Check sheet for the modelled part. Datum: model origin and axes. Units: mm. Round coordinates to 2 decimals unless told otherwise and drop trailing zeros. Loops run counter-clockwise (first coordinate to the right, second up) from the corner with the lowest first, then second, coordinate; pieces in that order, holes last. Notation, with made-up numbers: (5.5, -26) - (54.5, -26) arc R24 ccw to (54.5, 6) - close; hole circle Ø2 at (10.5, 38). An arc over 180 degrees is marked (long way). Put each result on its own line as item: value. Start each with the question number.
Item 1: Section check D-D, the plane y = -55.5. Record the cut outline in (x, z).
Item 2: Section check C-C, the plane x = 46.5. Record the cut outline in (y, z).
Item 3: Material ranges on line 1 along X through (y, z) = (105, 1.3); line 2 along Y through (x, z) = (46.5, 1.7); line 3 along X through (y, z) = (104, 2.5), recorded low to high.
Item 4: Section check B-B, the plane y = 45. Record the cut outline in (x, z), and give its area (3 significant figures).
Item 5: Section check A-A, the plane z = 4.1. Record the cut outline in (x, y).
Item 6: Gauge pin test, flat ends, axial feed: pin 1 Ø3 at (y, z) = (159, 1.5) entering from +X; pin 2 Ø2 at (y, z) = (-122.5, 5) entering from +X. Record the tip position at first contact, or that the pin passes through.
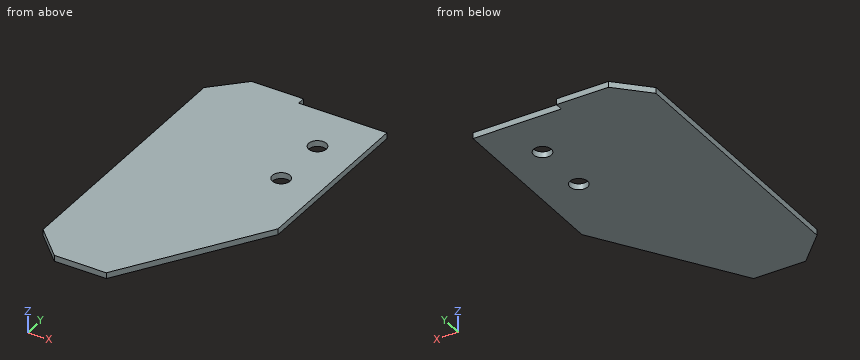
Autodesk Fusion 360 part; units mm, degrees
sketch "スケッチ1" plane through (0, 0, 0) normal (0, 0, 1) x (1, 0, 0)
  line L0 (-3.5, 163) -> (-86.5, 163)
  line L1 (-86.5, 163) -> (-86.5, -163)
  line L2 (-86.5, -163) -> (-3.5, -163)
  line L3 (86.5, -25) -> (86.5, 155)
  line L4 (82.2546, 155) -> (-86.5, -163) construction
  line L5 (-86.5, 163) -> (46.1223, -86.9125) construction
  line L6 (-3.5, 163) -> (-3.5, 155)
  line L7 (-3.5, 155) -> (86.5, 155)
  line L8 (-86.5, -163) -> (-3.5, -163) construction
  line L9 (86.5, -25) -> (-3.5, -163)
  dimension "d2" = 326
  dimension "d5" = 83
extrude "押し出し1" add sketch "スケッチ1" along normal blind 6
chamfer "面取り1" distance 30 angle 45 2 edges at (-86.5, -163, 3) (-86.5, 163, 3)
sketch "スケッチ2" plane through (0, 0, 6) normal (0, 0, 1) x (-1, 0, 0)
  line L0 (56.5, -163) -> (86.5, -133)
  line L1 (86.5, -133) -> (86.5, 133)
  line L2 (86.5, 133) -> (56.5, 163)
  line L3 (56.5, 163) -> (3.5, 163)
  line L4 (3.5, 163) -> (-86.5, 25)
  line L5 (-86.5, 25) -> (-86.5, -155)
  line L6 (-86.5, -155) -> (3.5, -155)
  line L7 (3.5, -155) -> (3.5, -163)
  line L8 (3.5, -163) -> (56.5, -163)
  line L9 (-86.5, -155) -> (-46.5, -155) construction
  line L10 (-46.5, -155) -> (-46.5, -105) construction
  line L11 (-46.5, -105) -> (-86.5, -105) construction
  line L12 (-86.5, -105) -> (-86.5, -155) construction
  line L13 (-46.5, -105) -> (-46.5, -45) construction
  point P0 (-46.5, -105)
  point P1 (-46.5, -45)
  dimension "d10" = 40
  dimension "d11" = 50
  dimension "d12" = 60
hole "穴1" at (46.5, 105, 6) at (46.5, 45, 6) direction (0, 0, -1) diameter 18 end through all
equation "d5 = 30 mm + 53 mm"
Check result:
1. outline: (-86.5, 0) - (66.61, 0) - (66.61, 6) - (-86.5, 6) - close
2. outline: (-86.33, 0) - (36, 0) - (36, 6) - (-86.33, 6) - close; (54, 0) - (96, 0) - (96, 6) - (54, 6) - close; (114, 0) - (155, 0) - (155, 6) - (114, 6) - close
3. line 1: -86.5 to 37.5, 55.5 to 86.5
3. line 2: -86.33 to 36, 54 to 96, 114 to 155
3. line 3: -86.5 to 37.56, 55.44 to 86.5
4. outline: (-86.5, 0) - (37.5, 0) - (37.5, 6) - (-86.5, 6) - close; (55.5, 0) - (86.5, 0) - (86.5, 6) - (55.5, 6) - close
4. area: 930 mm²
5. outline: (-86.5, -133) - (-56.5, -163) - (-3.5, -163) - (86.5, -25) - (86.5, 155) - (-3.5, 155) - (-3.5, 163) - (-56.5, 163) - (-86.5, 133) - close; hole circle Ø18 at (46.5, 45); hole circle Ø18 at (46.5, 105)
6. pin 1: x = -3.5
6. pin 2: x = 23.57
